Read the model definition and answer for the solid it produces. Units are mm, in the model's axes. A direction names the side the tool comes from. Give positions to 0.01 mm unless a question says otherwise; leave off trailing zeros. Order: outer loops, then holes, each group sorted by start corner. A loop starts at its lowest first (then second) coordinate and runs counter-clockwise, first axis right, second up.
Item 1: A cutting plane is placed at D-D (x = -10.5). Write down the section's boundary in (y, z), plus the area to 3 significant figures.
Item 2: Which of the six approach directions +Z, -Z, +X, -X, +Y, -Y give full straight-line access (tool end or side, diameter ignored) to faces 4 (the face through (-18.145, 21.143, -5.151)), 5 (the face through (-0.27, 1.96, 1.93))?
Item 3: A cutting plane is placed at C-C (y = -10). Write down the section's boundary in (x, z).
Item 4: A cutting plane is placed at B-B (x = 0). Write down the section's boundary in (y, z), plus the area to 3 significant figures.
Item 5: Given pin 1 Ø4 at (x, z) = (0.5, 1.5) entering from +Y; pin 2 Ø2 at (x, y) = (8.5, 17) entering from +Z; pin 3 Ø1.3 at (y, z) = (-1, 1) entering from -X, each flat-ended and moving along its own axis, determine where each tip first touches the part or whether it passes through.
Item 6: Find the intervals of material crossed by line 1 along Y through (x, z) = (0, 1.5); line 2 along Z through (x, y) = (-8, 16); line 3 along Y through (x, z) = (-5, 2.75), in increasing order.
Item 7: A cutting plane is placed at A-A (z = 0.75). State how many separate pieces and enclosed holes the cut face has, plus the area to 3 significant figures.
Item 8: The mould has two halves that part along X. Classify faces 1 (the face through (0, -22.098, -5)), 2 (the face through (3.92, -3.17, 1.93)), 3 (the face through (-19.05, 0, -5)): +X half, -X half, draft (parallel to the pull), parting line (faces both ways), or undercut.
Autodesk Inventor part; units mm, degrees
ref_plane "YZ Plane" through (0, 0, 0) normal (1, 0, 0) x (0, 1, 0)
ref_plane "XZ Plane" through (0, 0, 0) normal (0, 1, 0) x (-1, 0, 0)
ref_plane "XY Plane" through (0, 0, 0) normal (0, 0, 1) x (1, 0, 0)
sketch "FishmanBattery" plane through (0, 0, 0) normal (0, 0, 1) x (1, 0, 0)
  line L0 (-19.05, 22.098) -> (19.05, 22.098)
  line L1 (19.05, 22.098) -> (19.05, -22.098)
  line L2 (19.05, -22.098) -> (-19.05, -22.098)
  line L3 (-19.05, -22.098) -> (-19.05, 22.098)
  circle A0 centre (0, 0) radius 6.35
  line L4 (0, 22.098) -> (0, -22.098) construction
  line L5 (-19.05, 0) -> (19.05, 0) construction
  point P0 (0, 0)
  point P1 (0, 0)
  dimension "d13" = 38.1
  dimension "d14" = 44.196
  dimension "d26" = 12.7
extrude "FishmanBatteryFeature" add sketch "FishmanBattery" against normal blind 10.16 contours L0 L1 L2 L3 | A0
extrude "FishmanBatteryConnectorFeature" add sketch "FishmanBattery" along normal blind 3.81 contours A0
chamfer "FishmanBatteryChamferFeature" distance 0.381 angle 45 1 edges at (-6.35, 0, 3.81)
fillet "FishmanBatteryFilletsFeature" radius 3.175 4 edges at (19.05, 22.098, -5.08) (19.05, -22.098, -5.08) (-19.05, -22.098, -5.08) (-19.05, 22.098, -5.08)
sketch "FishmanConnector" plane through (0, 0, 3.81) normal (0, 0, 1) x (1, 0, 0)
  circle A0 centre (0, 3.175) radius 1.8791
  circle A1 centre (0, 3.175) radius 1.2441
  line L0 (-4.2333, 0) -> (4.2333, 0)
  line L1 (4.2333, 0) -> (4.2333, -2.6291)
  line L2 (4.2333, -2.6291) -> (3.5983, -3.729)
  line L3 (3.5983, -3.729) -> (-3.2605, -3.729)
  line L4 (-3.2605, -3.729) -> (-4.2333, -2.9126)
  line L5 (-4.2333, -2.9126) -> (-4.2333, 0)
  line L6 (0, -30.9372) -> (0, 30.9372) construction
  point P0 (0, 0)
  point P1 (0, 0)
  dimension "d133" = 3.729
  dimension "d134" = 8.4667
  dimension "d135" = 3.7582
  dimension "d136" = 0.635
  dimension "d137" = 150
  dimension "d138" = 140
  dimension "d139" = 1.27
  dimension "d141" = 3.175
extrude "FishmanConnectorHolesFeature" cut sketch "FishmanConnector" against normal blind 3.81
properties part number "fishman-battery"
Response values:
1. outline: (-22.1, -10.16) - (22.1, -10.16) - (22.1, 0) - (-22.1, 0) - close
1. area: 449 mm2
2. face 4: +Z, -Z, -X, +Y
2. face 5: +Z
3. outline: (-19.05, -10.16) - (19.05, -10.16) - (19.05, 0) - (-19.05, 0) - close
4. outline: (-22.1, -10.16) - (22.1, -10.16) - (22.1, 0) - (6.35, 0) - (6.35, 3.43) - (5.97, 3.81) - (5.05, 3.81) - (5.05, 0) - (4.42, 0) - (4.42, 3.81) - (1.93, 3.81) - (1.93, 0) - (1.3, 0) - (1.3, 3.81) - (0, 3.81) - (0, 0) - (-3.73, 0) - (-3.73, 3.81) - (-5.97, 3.81) - (-6.35, 3.43) - (-6.35, 0) - (-22.1, 0) - close
4. area: 478 mm2
5. pin 1: stops at y = 22.1
5. pin 2: stops at z = 0
5. pin 3: stops at x = -6.34
6. line 1: y = -6.35 to -3.73, 0 to 1.3, 1.93 to 4.42, 5.05 to 6.35
6. line 2: z = -10.16 to 0
6. line 3: y = -3.91 to 3.91
7. separate pieces: 2
7. enclosed holes: 2
7. area: 89.6 mm2
8. face 1: draft
8. face 2: undercut
8. face 3: -X half
